Can you work these out from the model? Positions are in its coordinate system, mm. Round coordinates to 2 decimals unless told otherwise and drop trailing zeros. Order: outer loops, then holes, each group sorted by start corner. A loop starts at its lowest first (then second) coordinate and runs counter-clockwise, first axis right, second up. Notation, with made-up numbers: (23.5, 21.25) -> (40.5, 21.25) arc R9 ccw to (40.5, 38.25) -> close; hole circle Ø10 at (-10, 65.5). An arc over 180 degrees is marked (long way). Use a Markdown table: item, result. Add a question column.
Q1. I'm going to push flat-ended pins straight in: pin 1 Ø4 at (y, z) = (-6.5, -4) entering from +X; pin 2 Ø8 at (x, y) = (-78, -9.5) entering from +Z (3 decimals); pin 3 Ø5 at (y, z) = (-6, 9) entering from -X. Where does each tip first touch, or does it pass through?
Q2. If we section it at A-A on z = 0: List the corners of the cut face in (x, y) for me, plus the area to 3 significant figures.
Q3. I need wall thicknesses on line 1 along Y through (x, z) = (-7.5, -0.5); line 2 along Z through (x, y) = (-92.5, -10); line 3 along Y through (x, z) = (-71.5, -7). Which ranges of each line are inside material? Lowest first, please. Write a range as [from, to].
Q4. If we section it at B-B on x = -15.5: List the corners of the cut face in (y, z) for me (3 decimals).
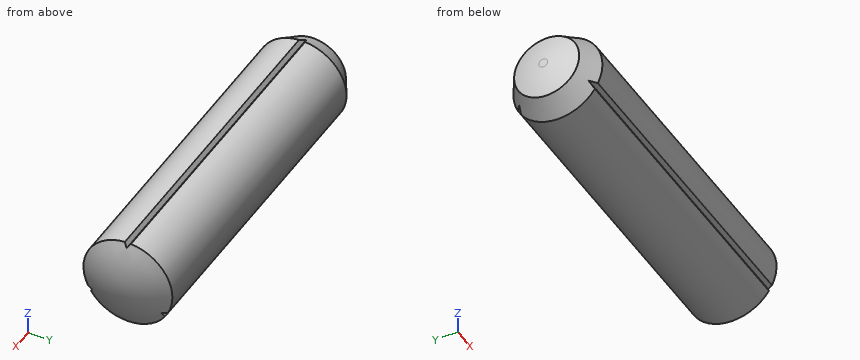
```python
from build123d import *

# Parameters (mm, degrees)
CUT_EXTRUDE1_DEPTH = 102.550480058
CIRPATTERN2_COUNT  = 3


with BuildPart() as part:
    # Sketch1 → Base-Revolve (revolve)
    with BuildSketch(Plane.XY):
        with BuildLine():
            Line((-92.5, 12.5), (-98.294957108, 9.154279954))
            ThreePointArc((-98.294957108, 9.154279954), (-99.46916936, 5.271532335), (-100, 1.25))
            Line((-100, 1.25), (-100, 0))
            Line((-100, 0), (0, 0))
            ThreePointArc((0, 0), (-0.851854343, 6.470476128), (-3.349364905, 12.5))
            Line((-3.349364905, 12.5), (-92.5, 12.5))
        make_face()
    revolve(axis=Axis((-117, 0, 0), (1, 0, 0)))

    # Sketch2 → Cut-Extrude1 (cut, through all)
    with BuildSketch(Plane(origin=(0, 0, 0), x_dir=(0, 0, -1), z_dir=(1, 0, 0))):
        Polygon((-11.25, 0), (-12.5, 0.875259423), (-12.5, -0.875259423), align=None)
    cut_extrude1 = extrude(amount=-CUT_EXTRUDE1_DEPTH, mode=Mode.SUBTRACT)

    # CirPattern2: Cut-Extrude1 ×3 about axis
    cirpattern2_axis = Axis((0, 0, 0), (1, 0, 0))
    for i in range(1, CIRPATTERN2_COUNT):
        add(cut_extrude1.rotate(cirpattern2_axis, i * 360 / CIRPATTERN2_COUNT), mode=Mode.SUBTRACT)


solid = part.part
```
Answer below:
| question | item | result |
|---|---|---|
| 1 | pin 1 | x = -0.64 |
| 1 | pin 2 | z = 11.225 |
| 1 | pin 3 | x = -98.61 |
| 2 | outline | (-100, -1.25) arc R25 ccw to (-98.29, -9.15) -> (-92.5, -12.5) -> (-3.35, -12.5) arc R25 ccw to (-3.35, 12.5) -> (-92.5, 12.5) -> (-98.29, 9.15) arc R25 ccw to (-100, 1.25) -> close |
| 2 | area | 2,430 mm² |
| 3 | line 1 | [-12.49, 12.49] |
| 3 | line 2 | [-7.5, -6.18], [-5.6, 7.5] |
| 3 | line 3 | [-10.36, 10.36] |
| 4 | outline | (-11.227, -5.495) -> (-9.743, -5.625) -> (-10.373, -6.976) arc R12.5 ccw to (10.373, -6.976) -> (9.743, -5.625) -> (11.227, -5.495) arc R12.5 ccw to (0.855, 12.471) -> (0, 11.25) -> (-0.855, 12.471) arc R12.5 ccw to start |
